```python
from build123d import *

# Parameters (mm, degrees)
F1_DEPTH = 25
F2_R     = 1.5875
F3_DEPTH = 25
F4_R     = 2.5
F5_DEPTH = 25


with BuildPart() as f1:
    # F0 (on Front) → F1 (new body)
    with BuildSketch(Plane.XZ):
        with BuildLine():
            Line((-17.3205080757, 10), (0, 0))
            Line((0, 0), (17.3205080757, 10))
            ThreePointArc((17.3205080757, 10), (0, 20), (-17.3205080757, 10))
        make_face()
        with BuildLine():
            ThreePointArc((19.918584287, 11.5), (0, 23), (-19.918584287, 11.5))
            Line((-19.918584287, 11.5), (-17.3205080757, 10))
            ThreePointArc((-17.3205080757, 10), (0, 20), (17.3205080757, 10))
            Line((17.3205080757, 10), (19.918584287, 11.5))
        make_face()
        with BuildLine():
            Line((19.3185165258, 5.1763809021), (22.2162940046, 5.9528380374))
            ThreePointArc((22.2162940046, 5.9528380374), (21.2492292478, 8.8017189444), (19.918584287, 11.5))
            Line((19.918584287, 11.5), (17.3205080757, 10))
            ThreePointArc((17.3205080757, 10), (18.4775906502, 7.6536686473), (19.3185165258, 5.1763809021))
        make_face()
        with BuildLine():
            Line((17.3205080757, 10), (0, 0))
            Line((0, 0), (19.3185165258, 5.1763809021))
            ThreePointArc((19.3185165258, 5.1763809021), (18.4775906502, 7.6536686473), (17.3205080757, 10))
        make_face()
        with BuildLine():
            Line((0, 0), (19.3185165258, -5.1763809021))
            ThreePointArc((19.3185165258, -5.1763809021), (19.8288972275, -2.6105238444), (20, 0))
            ThreePointArc((20, 0), (19.8288972275, 2.6105238444), (19.3185165258, 5.1763809021))
            Line((19.3185165258, 5.1763809021), (0, 0))
        make_face()
        with BuildLine():
            add(Edge.make_bspline(
                [(19.3185165258, -5.1763809021), (21.3890688866, 2.5510257083), (22.99275114, 3.0550605585), (22.2162940046, 5.9528380374)],
                knots=[0, 0, 0, 0, 11.5002881928, 11.5002881928, 11.5002881928, 11.5002881928], degree=3))
            Line((22.2162940046, 5.9528380374), (19.3185165258, 5.1763809021))
            ThreePointArc((19.3185165258, 5.1763809021), (19.8288972275, 2.6105238444), (20, 0))
            ThreePointArc((20, 0), (19.8288972275, -2.6105238444), (19.3185165258, -5.1763809021))
        make_face()
        with BuildLine():
            Line((0, 0), (17.3205080757, -10))
            ThreePointArc((17.3205080757, -10), (18.4775906502, -7.6536686473), (19.3185165258, -5.1763809021))
            Line((19.3185165258, -5.1763809021), (0, 0))
        make_face()
        with BuildLine():
            ThreePointArc((-17.3205080757, -10), (0, -20), (17.3205080757, -10))
            Line((17.3205080757, -10), (0, 0))
            Line((0, 0), (-17.3205080757, 10))
            ThreePointArc((-17.3205080757, 10), (-19.8288972275, 2.6105238444), (-19.3185165258, -5.1763809021))
            ThreePointArc((-19.3185165258, -5.1763809021), (-18.4775906502, -7.6536686473), (-17.3205080757, -10))
        make_face()
        with BuildLine():
            Line((-10, -40), (10, -40))
            add(Edge.make_bspline(
                [(12.9220055275, -19.0268697674), (10.9430027849, -24.3950055717), (10, -30.4378356334), (10, -40)],
                knots=[11.1947815786, 11.1947815786, 11.1947815786, 11.1947815786, 30.8802499745, 30.8802499745, 30.8802499745, 30.8802499745], degree=3))
            ThreePointArc((12.9220055275, -19.0268697674), (0, -23), (-12.9220055275, -19.0268697674))
            add(Edge.make_bspline(
                [(-12.9220055275, -19.0268697674), (-10.9430027849, -24.3950055717), (-10, -30.4378356334), (-10, -40)],
                knots=[11.1947815786, 11.1947815786, 11.1947815786, 11.1947815786, 30.8802499745, 30.8802499745, 30.8802499745, 30.8802499745], degree=3))
        make_face()
        with BuildLine():
            ThreePointArc((-12.9220055275, -19.0268697674), (0, -23), (12.9220055275, -19.0268697674))
            add(Edge.make_bspline(
                [(17.3205080757, -10), (15.5078961979, -13.1395358667), (14.0474297746, -15.9741048241), (12.9220055275, -19.0268697674)],
                knots=[0, 0, 0, 0, 11.1947815786, 11.1947815786, 11.1947815786, 11.1947815786], degree=3))
            ThreePointArc((17.3205080757, -10), (0, -20), (-17.3205080757, -10))
            add(Edge.make_bspline(
                [(-17.3205080757, -10), (-15.5078961979, -13.1395358667), (-14.0474297746, -15.9741048241), (-12.9220055275, -19.0268697674)],
                knots=[0, 0, 0, 0, 11.1947815786, 11.1947815786, 11.1947815786, 11.1947815786], degree=3))
        make_face()
        with BuildLine():
            ThreePointArc((-19.918584287, 11.5), (-21.2492292478, 8.8017189444), (-22.2162940046, 5.9528380374))
            add(Edge.make_bspline(
                [(-19.3185165258, -5.1763809021), (-21.3890688866, 2.5510257083), (-22.99275114, 3.0550605585), (-22.2162940046, 5.9528380374)],
                knots=[0, 0, 0, 0, 11.5002881928, 11.5002881928, 11.5002881928, 11.5002881928], degree=3))
            ThreePointArc((-19.3185165258, -5.1763809021), (-19.8288972275, 2.6105238444), (-17.3205080757, 10))
            Line((-17.3205080757, 10), (-19.918584287, 11.5))
        make_face()
    extrude(amount=F1_DEPTH)

    # F2 (on face) → F3 (cut)
    with BuildSketch(Plane.XZ.offset(25)):
        Circle(F2_R)
    extrude(amount=-F3_DEPTH, mode=Mode.SUBTRACT)

    # F4 (on face) → F5 (cut)
    with BuildSketch(Plane(origin=(0, 0, -40), x_dir=(1, 0, 0), z_dir=(0, 0, -1))):
        with Locations((0, 10)):
            Circle(F4_R)
    extrude(amount=-F5_DEPTH, mode=Mode.SUBTRACT)


solid = f1.part
```
For this review, take the finished solid that the model builds, in its own axes (mm). A direction names the side the tool comes from. Coordinates: 2 decimals unless noted, no trailing zeros. Loops run counter-clockwise (first coordinate to the right, second up) from the corner with the lowest first, then second, coordinate; pieces in that order, holes last. Notation, with made-up numbers: (23, -29.75) -> (73, -29.75) arc R30 ccw to (73, 5.25) -> close; hole circle Ø5 at (45, 75.5). An arc over 180 degrees is marked (long way). Return JSON: item names as keys, results as strings. Group by question number.
(1) To check wall thickness, follow L1, parallel to Y at x = 0, z = -34.5; L2, parallel to X at y = -10, z = -29; L3, parallel to X at y = -10, z = -30.5. State the ranges of each line that lie inside material, in increasing order.
(2) Consider section B-B, the plane z = 13. Give the boundary of the cut face in (x, y).
(3) Mouldability with a two-part tool opening along X and no side actions: class faces 3 (the cylindrical face through (-0.54, -7.56, -27.68)), 4 (the flat face through (0, 0, -8)), 5 (the cylindrical face through (18.464, -12.325, -7.688)) as pulls with the +X half, pulls with the -X half, needs draft (parallel to the pull), parting line crosses it, or undercut.
(4) For pin 1 Ø8 at (y, z) = (-13, -5) entering from -X; pin 2 Ø5 at (y, z) = (-3, 9.5) entering from +X; pin 3 Ø3 at (y, z) = (-11, 12.5) entering from +X, all flat-tipped, find the tip position at first contact; note any pin that passes through.
(5) Consider section A-A, the plane x = 0. Give the boundary of the cut face in (y, z), plus the area to 3 significant figures.
(6) Consider section C-C, the plane x = 9. Give the boundary of the cut face in (y, z), plus the area to 3 significant figures.
(7) Tool access review of faces 1 (the flat face through (0, -10, -15)), 2 (the flat face through (0, -25, -8)): name each direction out of +Z, -Z, +X, -X, +Y, -Y from which nothing blocks a thin tool from reaching the whole face with its end or side.
Results below:
{
 "1": {"L1": "y = -25 to -12.5, -7.5 to 0", "L2": "x = -10.58 to -2.5, 2.5 to 10.58", "L3": "x = -10.41 to -2.5, 2.5 to 10.41"},
 "2": {"outline": "(-18.97, -25) -> (18.97, -25) -> (18.97, 0) -> (-18.97, 0) -> close"},
 "3": {"face 3": "undercut", "face 4": "needs draft", "face 5": "pulls with the +X half"},
 "4": {"pin 1": "stops at x = -20.6", "pin 2": "stops at x = 21.91", "pin 3": "stops at x = 20.2"},
 "5": {"outline": "(-25, -40) -> (-12.5, -40) -> (-12.5, -15) -> (-7.5, -15) -> (-7.5, -40) -> (0, -40) -> (0, -1.59) -> (-25, -1.59) -> close; (-25, 1.59) -> (0, 1.59) -> (0, 23) -> (-25, 23) -> close", "area": "1,370 mm2"},
 "6": {"outline": "(-25, -40) -> (0, -40) -> (0, 21.17) -> (-25, 21.17) -> close", "area": "1,530 mm2"},
 "7": {"face 1": "-Z", "face 2": "+Z, -Z, +X, -X, -Y"}
}
